Autodesk Inventor part; units mm, degrees
ref_plane "Work Plane3" through (-48.921, -35.1, 35.161) normal (0, 0, 1) x (1, 0, 0)
ref_plane "YZ Plane" through (0, 0, 0) normal (1, 0, 0) x (0, 1, 0)
ref_plane "XZ Plane" through (0, 0, 0) normal (0, 1, 0) x (-1, 0, 0)
ref_plane "Work Plane1" through (0, 0, 0) normal (0, 0, 1) x (1, 0, 0)
ref_plane "Work Plane2" through (0, 0, 0) normal (0, 0, 1) x (1, 0, 0)
sketch "Sketch2" plane through (0, 0, 0) normal (0, 0, 1) x (1, 0, 0)
  circle A0 centre (44.9, -55.1) radius 1.6 construction
  circle A1 centre (44.9, -45.1) radius 1.6 construction
  line L0 (49.9, -97.9) -> (49.9, 41.0746) construction
  line L1 (-49.9, -35.1) -> (-49.9, -97.9) construction
  circle A2 centre (-45.1, -45.1) radius 1.6 construction
  circle A3 centre (-45.1, -55.1) radius 1.4 construction
  line L2 (-2.8791, -35.1) -> (-48.921, -35.1) construction
  circle A4 centre (44.9, -5.1) radius 1.6 construction
  circle A5 centre (44.9, 4.9) radius 1.6 construction
  line L3 (49.9, -58.5557) -> (41.9, -58.5557) construction
  line L4 (41.9, -58.5557) -> (41.9, 19.8666) construction
  line L5 (41.9, 19.8666) -> (49.9, 19.8666) construction
  line L6 (49.9, 19.8666) -> (49.9, -58.5557) construction
  line L7 (41.9, -58.5557) -> (49.9, -58.5557)
  line L8 (49.9, -58.5557) -> (49.9, 19.8666)
  line L9 (49.9, 19.8666) -> (41.9, 19.8666)
  line L10 (41.9, 19.8666) -> (41.9, -58.5557)
  line L11 (41.9, 19.8666) -> (49.9, 36.639)
  line L12 (49.9, 19.8666) -> (49.9, 36.639)
  line L13 (60.4304, 64.9211) -> (17.3793, -25.3374)
  line L14 (-49.9, -58.0504) -> (-41.9, -58.0504)
  line L15 (-41.9, -58.0504) -> (-41.9, -38.0504)
  line L16 (-41.9, -38.0504) -> (-49.9, -38.0504)
  line L17 (-49.9, -38.0504) -> (-49.9, -58.0504)
  line L18 (-41.9, -58.0504) -> (-39.9, -58.0504)
  line L19 (-39.9, -58.0504) -> (-39.9, -38.0504)
  line L20 (-39.9, -38.0504) -> (-41.9, -38.0504)
  line L21 (-41.9, -38.0504) -> (-41.9, -58.0504)
  line L22 (41.9, -58.5557) -> (39.9, -58.5557)
  line L23 (39.9, -58.5557) -> (39.9, 19.7918)
  line L24 (39.9, 19.7918) -> (41.9, 19.7918)
  line L25 (41.9, 19.7918) -> (41.9, -58.5557)
  circle A6 centre (-45.1, -55.1) radius 1.4
  circle A7 centre (-45.1, -45.1) radius 1.6
  circle A8 centre (44.9, -55.1) radius 1.6
  circle A9 centre (44.9, -45.1) radius 1.6
  circle A10 centre (44.9, -5.1) radius 1.6
  circle A11 centre (44.9, 4.9) radius 1.6
  line L26 (39.9, -58.5557) -> (9.9, -58.5557)
  line L27 (9.9, -58.5557) -> (9.9, -56.5557)
  line L28 (9.9, -56.5557) -> (39.9, -56.5557)
  line L29 (39.9, -56.5557) -> (39.9, -58.5557)
  point P0 (0, 0)
  dimension "d0" = 8
  dimension "d1" = 8
  dimension "d2" = 20
  dimension "d3" = 2
  dimension "d4" = 2
  dimension "d7" = 30
  dimension "d8" = 2
extrude "Extrusion1" add sketch "Sketch2" along normal blind 2 contours L10 L9 L8 L7 | L22 L23 L24 L10 | L26 L27 L28 L23 | L17 L16 L15 L14 | L15 L20 L19 L18
sketch "Sketch3" plane through (0, 0, 2) normal (0, 0, 1) x (1, 0, 0)
  line L0 (39.9, 19.7918) -> (39.9, -56.5557)
  circle A0 centre (44.9, 4.9) radius 1.6
  circle A1 centre (44.9, -5.1) radius 1.6
  circle A2 centre (44.9, -45.1) radius 1.6
  circle A3 centre (44.9, -55.1) radius 1.6
  line L1 (39.9, -56.5557) -> (9.9, -56.5557)
  line L2 (9.9, -56.5557) -> (9.9, -58.5557)
  line L3 (9.9, -58.5557) -> (49.9, -58.5557)
  line L4 (49.9, -58.5557) -> (49.9, 19.8666)
  line L5 (49.9, 19.8666) -> (41.9, 19.8666)
  line L6 (41.9, 19.8666) -> (41.9, 19.7918)
  line L7 (41.9, 19.7918) -> (39.9, 19.7918)
  line L8 (39.9, 19.7918) -> (39.9, -56.5557)
  line L9 (39.9, 19.7918) -> (39.9, -56.5557)
  line L10 (9.9, -58.5557) -> (49.9, -58.5557)
  line L11 (39.9, 19.7918) -> (41.9, 19.7918)
  line L12 (41.9, 19.7918) -> (41.9, -58.5557)
  line L13 (41.9, -58.5557) -> (39.9, -58.5557)
  line L14 (39.9, -58.5557) -> (39.9, 19.7918)
  line L15 (39.9, -56.5557) -> (9.9, -56.5557)
  line L16 (9.9, -58.5557) -> (39.9, -58.5557)
  line L17 (39.9, -58.5557) -> (39.9, -56.5557)
  line L18 (39.9, -56.5557) -> (9.9, -56.5557)
  line L19 (9.9, -56.5557) -> (9.9, -58.5557)
  line L20 (-39.9, -58.0504) -> (-39.9, -38.0504)
  line L21 (-49.9, -58.0504) -> (-39.9, -58.0504)
  line L22 (-39.9, -38.0504) -> (-41.9, -38.0504)
  line L23 (-41.9, -38.0504) -> (-41.9, -58.0504)
  line L24 (-41.9, -58.0504) -> (-39.9, -58.0504)
  line L25 (-39.9, -58.0504) -> (-39.9, -38.0504)
  point P0 (0, 0)
  dimension "d9" = 2
ref_plane "Work Plane3" through (-48.921, -35.1, 35.161) normal (0, 0, 1) x (1, 0, 0)
extrude "Extrusion2" add sketch "Sketch3" along normal up to surface (33.161 mm away) contours L7 L12 L3 L14 L0 | L14 L3 L2 L1 | L21 L23 L22 L20
sketch "Sketch5" plane through (9.9, -58.5557, 35.161) normal (0, 0, 1) x (1, 0, 0)
  line L0 (0, 0) -> (0, 2)
  line L1 (32, 0) -> (0, 0)
  line L2 (32, 78.3475) -> (32, 0)
  line L3 (30, 78.3475) -> (32, 78.3475)
  line L4 (30, 2) -> (30, 78.3475)
  line L5 (0, 2) -> (30, 2)
  line L6 (-49.8, 20.5053) -> (-49.8, 0.5053)
  line L7 (-51.8, 20.5053) -> (-49.8, 20.5053)
  line L8 (-51.8, 0.5053) -> (-51.8, 20.5053)
  line L9 (-49.8, 0.5053) -> (-51.8, 0.5053)
  line L10 (32, 78.3475) -> (-51.8, 78.3475)
  line L11 (-51.8, 78.3475) -> (-51.8, 0.5053)
  line L12 (-51.8, 0.5053) -> (32, 0.5053)
  line L13 (32, 0.5053) -> (32, 78.3475)
  line L14 (32, 78.3475) -> (32, 0)
  line L15 (32, 0) -> (-51.8, 0)
  line L16 (-51.8, 0) -> (-51.8, 0.5053)
  line L17 (-51.8, 0.5053) -> (32, 0.5053)
  line L18 (32, 0.5053) -> (32, 0)
  point P0 (-9.9, 58.5557)
extrude "Extrusion3" add sketch "Sketch5" along normal blind 2
sketch "Sketch6" plane through (-41.9, -58.0504, 2) normal (-1, 0, 0) x (0, 0, 1)
  line L0 (0, 20) -> (33.161, 20)
  line L1 (0, 0) -> (0, 20)
  line L2 (0, 0) -> (33.161, 0)
  line L3 (33.161, 0) -> (33.161, -0.5053)
  line L4 (33.161, -0.5053) -> (35.161, -0.5053)
  line L5 (35.161, 77.8423) -> (35.161, -0.5053)
  line L6 (33.161, 77.8423) -> (35.161, 77.8423)
  line L7 (33.161, 77.8423) -> (33.161, 20)
  line L8 (-2, 7.7504) -> (-2, -86.2156)
  line L9 (-2, -86.2156) -> (3, -86.2156)
  line L10 (3, -19.7496) -> (3, -86.2156)
  line L11 (3, -19.7496) -> (7.1792, -19.7496)
  line L12 (7.1792, -19.7496) -> (7.1792, -14.7496)
  line L13 (3, -14.7496) -> (7.1792, -14.7496)
  line L14 (3, 7.7504) -> (3, -14.7496)
  line L15 (-2, 7.7504) -> (3, 7.7504)
  line L16 (-2.5429, 8.2795) -> (3.9802, 8.2795)
  line L17 (3.9802, 8.2795) -> (3.9802, -0.9887)
  line L18 (3.9802, -0.9887) -> (-2.5429, -0.9887)
  line L19 (-2.5429, -0.9887) -> (-2.5429, 8.2795)
  point P0 (-2, 58.0504)
extrude "Extrusion4" cut sketch "Sketch6" along normal mid plane 20 contours L16 L17 L2 L14 L15 L1 | L1 L15 L8 L18 L19 L16 | L15 L14 L2 L1 | L1 L2 L14 L18 L8 L15 | L17 L18 L14 L2
properties part number "30_CUBE_openSIM_Lasershield"
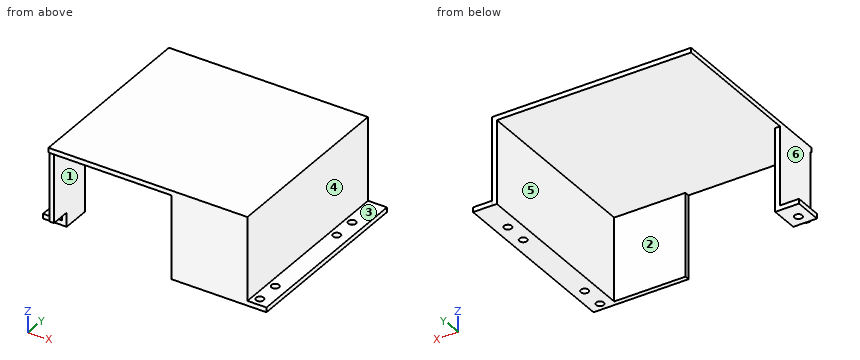
Geometry: final body of the model. Coordinates: model frame, mm. Face numbers are marked on the shaded views. A direction names the side the tool comes from. Give positions to 0.01 mm unless a question says otherwise; leave off trailing zeros. Order: outer loops, then holes, each group sorted by start corner. A loop starts at its lowest first (then second) coordinate and runs counter-clockwise, first axis right, second up. Notation, with made-up numbers: (47.25, 33) -> (82.25, 33) arc R19 ccw to (82.25, 62) -> close; hole circle Ø1 at (53, 83.5). An arc over 180 degrees is marked (long way). Write each question's results on one line, items separated by ' | '.
1) Cut plane D-D (x = -36.5). Output: boundary loops of the cut face in (y, z), and give its area (3 significant figures).
Geometry says:
outline: (-58.56, 35.16) -> (19.79, 35.16) -> (19.79, 37.16) -> (-58.56, 37.16) -> close | area: 157 mm²
2) Line query: line 1 along Y through (x, z) = (44.9, 1.1); line 2 along X through (y, z) = (-40, 11.5); line 3 along Y through (x, z) = (-45.1, 1). Output: solid intervals per line, ascending.
Geometry says:
line 1: y = -58.56 to -56.7, -53.5 to -46.7, -43.5 to -6.7, -3.5 to 3.3, 6.5 to 19.87 | line 2: x = -41.9 to -39.9, 39.9 to 41.9 | line 3: y = -49.77 to -46.7, -43.5 to -38.05
3) Draft query along X for the marked faces 4, 5 and 6. Return one class per face: released by +X, released by -X, zero draft, split by the parting line, or undercut.
Geometry says:
face 4: released by +X | face 5: undercut | face 6: released by -X
4) Set-up query: the marked faces 1, 2 and 3. Return all of +Z, -Z, +X, -X, +Y, -Y with unobstructed straight access to the full face (end or side cutting, diameter ignored); none if empty.
Geometry says:
face 1: -Z, +Y, -Y | face 2: -Z, +Y | face 3: +Z, +X, +Y, -Y
5) First-contact query: pin 1 Ø4 at (x, y) = (23.5, -11) entering from -Z; pin 2 Ø6 at (y, z) = (-43, 13.5) entering from +X; pin 3 Ø17.5 at (y, z) = (-32.5, 27) entering from -X; pin 4 Ø3 at (x, z) = (-45, 19.5) entering from +Y. Flat tips, straight axial feed; report the tip coordinate or a pass-through.
Geometry says:
pin 1: stops at z = 35.16 | pin 2: stops at x = 41.9 | pin 3: stops at x = -41.9 | pin 4: passes through
6) Cut plane C-C (y = -45.1). Output: boundary loops of the cut face in (x, z), and give its area (3 significant figures).
Geometry says:
outline: (-49.9, 0) -> (-46.7, 0) -> (-46.7, 2) -> (-49.9, 2) -> close; (-43.5, 0) -> (-39.9, 0) -> (-39.9, 35.16) -> (39.9, 35.16) -> (39.9, 0) -> (43.3, 0) -> (43.3, 2) -> (41.9, 2) -> (41.9, 37.16) -> (-41.9, 37.16) -> (-41.9, 2) -> (-43.5, 2) -> close; (46.5, 0) -> (49.9, 0) -> (49.9, 2) -> (46.5, 2) -> close | area: 327 mm²
7) Cut plane A-A (y = -55.1). Output: boundary loops of the cut face in (x, z), and give its area (3 significant figures).
Geometry says:
outline: (-41.9, 5.98) -> (-39.9, 5.98) -> (-39.9, 35.16) -> (39.9, 35.16) -> (39.9, 0) -> (43.3, 0) -> (43.3, 2) -> (41.9, 2) -> (41.9, 37.16) -> (-41.9, 37.16) -> close; (46.5, 0) -> (49.9, 0) -> (49.9, 2) -> (46.5, 2) -> close | area: 306 mm²
8) Cut plane B-B (z = 8). Output: boundary loops of the cut face in (x, y).
Geometry says:
outline: (-41.9, -58.05) -> (-39.9, -58.05) -> (-39.9, -38.05) -> (-41.9, -38.05) -> close; (9.9, -58.56) -> (41.9, -58.56) -> (41.9, 19.79) -> (39.9, 19.79) -> (39.9, -56.56) -> (9.9, -56.56) -> close
